Can you work these out from the model? Positions are in its coordinate system, mm. Coordinates: 2 decimals unless noted, no trailing zeros. Order: outer loops, then holes, each group sorted by start corner. A loop starts at its lowest first (then second) coordinate and runs counter-clockwise, first axis right, second up. Notation, with made-up numbers: (15.5, 40.25) -> (28.5, 40.25) arc R33 cw to (28.5, 70.25) -> close; hole circle Ø7 at (68.5, 67). An arc over 180 degrees is marked (long way). Answer in a Markdown table with one row per item. Add a question column.
1. Imagine slicing it at B-B on y = 27.5. Write out the boundary of the cut face in (x, z) (3 decimals).
2. Imagine slicing it at D-D on x = 38.5. Write out the boundary of the cut face in (y, z) (3 decimals), plus the area to 3 significant figures.
3. Imagine slicing it at A-A on x = 55. Write out the boundary of the cut face in (y, z) (3 decimals), plus the area to 3 significant figures.
4. If I drill on line 1 along Y through (x, z) = (-19, 1.7); line 2 along Y through (x, z) = (49, 0.4); line 3 along Y through (x, z) = (37, 0.85), over which ranges is the centre line in solid material (lowest first)? Write a range as [from, to].
5. Will these pins go through, and if not, where does the flat tip stop? pin 1 (1 mm diameter, centred on y = 27, z = 0.5, fed in from -X); pin 2 (2.5 mm diameter, centred on x = -19.11, y = 11.66, fed in from -Z).
6. Imagine slicing it at C-C on z = 0.55. State how many separate pieces and enclosed holes the cut face has, plus the area to 3 significant figures.
Autodesk Inventor part; units mm, degrees
ref_plane "YZ Plane" through (0, 0, 0) normal (1, 0, 0) x (0, 1, 0)
ref_plane "XZ Plane" through (0, 0, 0) normal (0, 1, 0) x (-1, 0, 0)
ref_plane "XY Plane" through (0, 0, 0) normal (0, 0, 1) x (1, 0, 0)
sketch "Sketch1" plane through (0, 0, 0) normal (0, 0, 1) x (1, 0, 0)
  arc A0 (-0.0635, 21.727) -> (-1.9234, 26.2171) centre (-6.4135, 21.727) ccw
  line L0 (-12.7635, 37.0572) -> (-1.9234, 26.2171)
  arc A1 (-12.7635, 37.0572) -> (-22.9837, 35.3037) centre (-17.2536, 32.5671) ccw
  arc A2 (-22.9837, 35.3037) -> (-25.4635, 24.3572) centre (-0.0635, 24.3572) ccw
  line L1 (-25.4635, 8.4822) -> (-25.4635, 24.3572)
  arc A3 (-25.4635, 8.4822) -> (-20.3429, -6.8118) centre (-0.0635, 8.4822) ccw
  line L2 (2.6238, -37.2648) -> (-20.3429, -6.8118)
  arc A4 (2.6238, -37.2648) -> (22.9032, -21.9707) centre (12.7635, -29.6178) ccw
  line L3 (1.2167, 6.7848) -> (22.9032, -21.9707)
  arc A5 (-0.0635, 10.6083) -> (1.2167, 6.7848) centre (6.2865, 10.6083) ccw
  line L4 (-0.0635, 21.727) -> (-0.0635, 10.6083)
  circle A6 centre (-19.1135, 24.3572) radius 2.159
  circle A7 centre (-6.4135, 24.3572) radius 2.159
  circle A8 centre (-6.4135, -13.7428) radius 2.159
  circle A9 centre (-6.4135, -1.0428) radius 2.159
  circle A10 centre (-6.4135, 11.6572) radius 2.159
  circle A11 centre (-19.1135, 11.6572) radius 2.159
  circle A12 centre (12.7635, -29.6178) radius 2.159
  line L5 (81.8636, -46.7367) -> (81.8636, 125.7735) construction
  line L6 (61.5605, 6.4848) -> (81.5605, 6.4848) construction
  line L7 (81.5605, 6.4848) -> (81.5605, 146.4848) construction
  line L8 (81.5605, 146.4848) -> (61.5605, 146.4848) construction
  line L9 (61.5605, 146.4848) -> (61.5605, 6.4848) construction
  circle A13 centre (53.9115, 41.9458) radius 25.4 construction
  arc A14 (49.9598, 13.7707) -> (6.7541, 27.2154) centre (12.7635, -29.6178) ccw construction
  arc A15 (53.9115, 41.9458) -> (38.0365, 48.9684) centre (12.7635, -29.6178) ccw construction
  arc A16 (57.0767, 47.4507) -> (39.9806, 55.0134) centre (12.7635, -29.6178) ccw
  arc A17 (50.7463, 36.4409) -> (36.0924, 42.9233) centre (12.7635, -29.6178) ccw
  arc A18 (50.7463, 36.4409) -> (57.0767, 47.4507) centre (53.9115, 41.9458) ccw
  arc A19 (39.9806, 55.0134) -> (36.0924, 42.9233) centre (38.0365, 48.9684) ccw
  circle A20 centre (38.0365, 48.9684) radius 25.4 construction
  arc A21 (53.9115, 41.9458) -> (38.0365, 48.9684) centre (12.7635, -29.6178) ccw construction
  arc A22 (60.242, 52.9556) -> (41.9247, 61.0585) centre (12.7635, -29.6178) ccw construction
  arc A23 (47.581, 30.936) -> (34.1483, 36.8782) centre (12.7635, -29.6178) ccw construction
  arc A24 (47.581, 30.936) -> (60.242, 52.9556) centre (53.9115, 41.9458) ccw
  arc A25 (41.9247, 61.0585) -> (34.1483, 36.8782) centre (38.0365, 48.9684) ccw construction
  circle A26 centre (-19.1135, 11.6572) radius 6.35
  circle A27 centre (-6.4135, 11.6572) radius 6.35
  line L10 (-6.4135, 5.3072) -> (-19.1135, 5.3072)
  line L11 (-0.0635, 21.727) -> (-0.0635, 24.3572)
  arc A28 (47.581, 30.936) -> (34.1483, 36.8782) centre (12.7635, -29.6178) ccw construction
  arc A29 (48.6572, 32.8077) -> (34.8093, 38.9335) centre (12.7635, -29.6178) ccw
  arc A30 (46.5049, 29.0644) -> (33.4874, 34.8229) centre (12.7635, -29.6178) ccw
  arc A31 (46.5049, 29.0644) -> (48.6572, 32.8077) centre (47.581, 30.936) ccw
  arc A32 (34.8093, 38.9335) -> (33.4874, 34.8229) centre (34.1483, 36.8782) ccw
  line L12 (38.0365, 48.9684) -> (12.7635, -29.6178) construction
  line L13 (53.9115, 41.9458) -> (12.7635, -29.6178) construction
  arc A33 (60.242, 52.9556) -> (41.9247, 61.0585) centre (12.7635, -29.6178) ccw construction
  arc A34 (61.3181, 54.8273) -> (42.5856, 63.1139) centre (12.7635, -29.6178) ccw
  arc A35 (59.1658, 51.0839) -> (41.2637, 59.0032) centre (12.7635, -29.6178) ccw
  arc A36 (59.1658, 51.0839) -> (61.3181, 54.8273) centre (60.242, 52.9556) ccw
  arc A37 (42.5856, 63.1139) -> (41.2637, 59.0032) centre (41.9247, 61.0585) ccw
  line L14 (38.0365, 48.9684) -> (41.9247, 61.0585) construction
  arc A38 (56.0006, 45.579) -> (39.3196, 52.9581) centre (12.7635, -29.6178) ccw
  arc A39 (56.0006, 45.579) -> (64.4834, 60.3321) centre (60.242, 52.9556) ccw
  arc A40 (64.4834, 60.3321) -> (44.5297, 69.1589) centre (12.7635, -29.6178) ccw
  arc A41 (44.5297, 69.1589) -> (39.3196, 52.9581) centre (41.9247, 61.0585) ccw
  arc A42 (51.8224, 38.3126) -> (36.7534, 44.9786) centre (12.7635, -29.6178) ccw
  arc A43 (36.7534, 44.9786) -> (31.5433, 28.7778) centre (34.1483, 36.8782) ccw
  arc A44 (43.3396, 23.5595) -> (31.5433, 28.7778) centre (12.7635, -29.6178) ccw
  arc A45 (43.3396, 23.5595) -> (51.8224, 38.3126) centre (47.581, 30.936) ccw
  line L15 (62.2155, 32.3368) -> (53.1447, 24.498)
  line L16 (66.3936, 39.6032) -> (68.605, 51.386)
  line L17 (34.4081, 61.139) -> (-7.3204, 48.6985)
  arc A46 (-7.3204, 48.6985) -> (-22.9837, 35.3037) centre (-0.0635, 24.3572) ccw
  line L18 (-0.0635, 24.3572) -> (37.7202, 35.6217)
  point P0 (0, 0)
  point P1 (-0.0635, 11.6572)
  point P2 (-25.4635, 11.6572)
  point P3 (-12.7635, 11.6572)
  point P4 (33.4184, 60.8439)
  point P5 (26.9132, 32.3998)
  dimension "d0" = 20
  dimension "d1" = 140
  dimension "d2" = 50.8
  dimension "d3" = 57.15
  dimension "d4" = 53.975
  dimension "d6" = 12.7
  dimension "d7" = 38.1
  dimension "d8" = 25.4
  dimension "d11" = 4.318
  dimension "d12" = 12.7
  dimension "d13" = 12.7
  dimension "d14" = 6.35
  dimension "d15" = 6.35
extrude "Extrusion1" add sketch "Sketch1" along normal blind 3.175 contours L4 A27 A26 L1 A2 A1 L0 A0 | A0 L0 A1 A46 L17 A41 A19 A43 L18 L11 | A27 | A27 L10 A26 | A26 | L18 A30 A31 A24 A45 A44 A43 | A43 A19 A17 A18 A45 A24 A31 A29 A32 A30 L18 | A41 A40 A39 A18 A16 A19 | A45 A24 L15 | A18 A39 A24 A45 | A24 A39 L16
fillet "Fillet1" radius 25.4 2 edges at (26.9132, 32.3998, 1.5875) (33.4184, 60.8439, 1.5875)
fillet "Fillet2" radius 3.175 1 edges at (-0.0635, 24.3572, 1.5875)
properties part number "IntakeForearm" material "Polycarbonate, Clear"
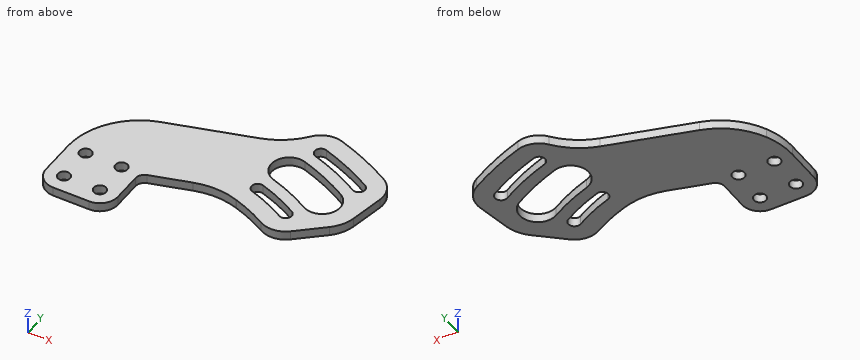
Answers follow:
| question | item | result |
|---|---|---|
| 1 | outline | (-25.268, 0) -> (10.478, 0) -> (10.478, 3.175) -> (-25.268, 3.175) -> close; (35.13, 0) -> (56.619, 0) -> (56.619, 3.175) -> (35.13, 3.175) -> close |
| 2 | outline | (26.063, 0) -> (32.99, 0) -> (32.99, 3.175) -> (26.063, 3.175) -> close; (37.635, 0) -> (42.104, 0) -> (42.104, 3.175) -> (37.635, 3.175) -> close; (55.301, 0) -> (68.848, 0) -> (68.848, 3.175) -> (55.301, 3.175) -> close |
| 2 | area | 79.2 mm² |
| 3 | outline | (26.101, 0) -> (35.69, 0) -> (35.69, 3.175) -> (26.101, 3.175) -> close; (48.608, 0) -> (53.34, 0) -> (53.34, 3.175) -> (48.608, 3.175) -> close; (58.158, 0) -> (65.156, 0) -> (65.156, 3.175) -> (58.158, 3.175) -> close |
| 3 | area | 67.7 mm² |
| 4 | line 1 | y = [5.31, 9.5], [13.81, 22.2], [26.51, 41.29] |
| 4 | line 2 | y = [22.55, 29.31], [32.56, 37.41], [51.56, 56.13], [60.8, 67.61] |
| 4 | line 3 | y = [26.73, 33.59], [38.19, 42.63], [55.23, 68] |
| 5 | pin 1 | stops at x = -25.37 |
| 5 | pin 2 | passes through |
| 6 | separate pieces | 1 |
| 6 | enclosed holes | 7 |
| 6 | area | 2,640 mm² |
